Verification items for the finished model (mm, model axes). A direction names the side the tool comes from. Give positions to 0.01 mm unless a question says otherwise; leave off trailing zeros. Write each loop counter-clockwise with the first axis right and the second up, starting at its lowest first coordinate (ties: lowest second). Pieces come first, ordered by that corner, then holes. Notation, with made-up numbers: (64, 34.5) -> (123, 34.5) arc R27 cw to (123, 59.5) -> close; hole circle Ø5 at (38.25, 64). An arc over 180 degrees is marked (long way). Use one line per item in the form item = value. Start each with the question number.
(1) Section check A-A, the plane x = -3.25. Record the cut outline in (y, z).
(2) Set-up check for faces 1 (the face through (-8.248, 11, -5)), 2 (the face through (2.692, -16.756, -3.409)), 3 (the face through (-11.187, -12.966, 1.479)): record each of +Z, -Z, +X, -X, +Y, -Y from which the full face is reachable in a straight line by a thin tool's end or side.
(3) Section check C-C, the plane y = 4.5. Record the cut outline in (x, z), plus the area to 3 significant figures.
(4) Depth check by flat-ended pin: pin 1 Ø1 at (x, y) = (-7, 57.5) entering from -Z; pin 2 Ø6.5 at (x, y) = (5.78, 63.88) entering from -Z; pin 3 Ø3 at (y, z) = (15.5, -3.5) entering from -X; pin 4 Ø3 at (y, z) = (0.5, -2.5) entering from +X. Enter the tip coordinate at first touch or a pass-through.
(5) Section check D-D, the plane z = 2. Record the cut outline in (x, y), plus the area to 3 significant figures.
(6) Section check B-B, the plane z = -4.5. Record the cut outline in (x, y), plus the area to 3 significant figures.
(7) Scan lines: L1, parallel to Z at x = -1, y = -17; L2, parallel to X at y = 3.5, z = -7.75; L3, parallel to X at y = -1.5, z = 1.75. Record each from-to range of solid material in increasing order.
(8) Release check for a two-part mould opening along X. For faces 4 (the face through (5.24, 61.44, 1.48)), 5 (the face through (-6.879, 10, -3)), 6 (the face through (1.24, -17.16, -4.93)), 7 (the face through (-4, -8, -10)) record: pulls with the +X half, pulls with the -X half, needs draft (parallel to the pull), parting line crosses it, or undercut.
from build123d import *

# Parameters (mm, degrees)
EXTRUDE_4_DEPTH     = 3
SKETCH_2_R          = 2.5
CUT_EXTRUDE_1_DEPTH = 72.936469634
EXTRUDE_6_DEPTH     = 10


with BuildPart() as part:
    # 草图1 → 凸台-拉伸4 (new body)
    with BuildSketch(Plane.XY):
        with BuildLine():
            ThreePointArc((11.999755772, 64.190702015), (7.19287537, 69.699227744), (0.441332655, 66.894477154))
            Line((0.441332655, 66.894477154), (-16.87917542, 36.894477154))
            Line((-16.87917542, 36.894477154), (-16.87917542, -3.105522846))
            Line((-16.87917542, -3.105522846), (-5.332170037, -23.105522846))
            Line((-5.332170037, -23.105522846), (9.992741519, -33.105522846))
            Line((9.992741519, -33.105522846), (11.999755772, -30.029791253))
            Line((11.999755772, -30.029791253), (-6.87917542, -3.105522846))
            Line((-6.87917542, -3.105522846), (-6.87917542, 14.190702015))
            Line((-6.87917542, 14.190702015), (-6.87917542, 24.190702015))
            Line((-6.87917542, 24.190702015), (10.114332844, 34.190702015))
            Line((10.114332844, 34.190702015), (11.999755772, 64.190702015))
        make_face()
    extrude(amount=EXTRUDE_4_DEPTH)

    # 草图2 → 切除-拉伸1 (cut, through all)
    with BuildSketch(Plane.XY):
        with Locations((5.784422652, 63.881230161)):
            Circle(SKETCH_2_R)
    extrude(amount=CUT_EXTRUDE_1_DEPTH, mode=Mode.SUBTRACT)

    # 草图6 → 凸台-拉伸6 (add)
    with BuildSketch(Plane(origin=(0, 0, 0), x_dir=(-1, 0, 0), z_dir=(0, 0, -1))):
        Polygon((6.87917542, 24.190702015), (8.248400541, 24.190702015), (8.248400541, -3.145484966), (-10.996248645, -31.567657049), (-11.999755772, -30.029791253), (6.87917542, -3.105522846), align=None)
    extrude(amount=EXTRUDE_6_DEPTH)


solid = part.part
Completed:
q1.outline = (-24.46, 0) -> (-10.53, 0) -> (-10.53, -10) -> (-8.28, -10) -> (-8.28, 3) -> (-24.46, 3) -> close; (26.33, 0) -> (60.5, 0) -> (60.5, 3) -> (26.33, 3) -> close
q2.face_1 = -Z, -X, +Y, -Y
q2.face_2 = +Z, -Z, +X
q2.face_3 = +Z, -Z, -X, -Y
q3.outline = (-16.88, 0) -> (-8.25, 0) -> (-8.25, -10) -> (-6.88, -10) -> (-6.88, 3) -> (-16.88, 3) -> close
q3.area = 43.7 mm²
q4.pin_1 = through
q4.pin_2 = 0
q4.pin_3 = -8.25
q4.pin_4 = -6.88
q5.outline = (-16.88, -3.11) -> (-5.33, -23.11) -> (9.99, -33.11) -> (12, -30.03) -> (-6.88, -3.11) -> (-6.88, 24.19) -> (10.11, 34.19) -> (12, 64.19) arc R6.26 ccw to (0.44, 66.89) -> (-16.88, 36.89) -> close; hole circle Ø5 at (5.78, 63.88)
q5.area = 1,420 mm²
q6.outline = (-8.25, -3.15) -> (11, -31.57) -> (12, -30.03) -> (-6.88, -3.11) -> (-6.88, 24.19) -> (-8.25, 24.19) -> close
q6.area = 85.3 mm²
q7.L1 = 0 to 3
q7.L2 = -8.25 to -6.88
q7.L3 = -16.88 to -6.88
q8.face_4 = undercut
q8.face_5 = pulls with the +X half
q8.face_6 = pulls with the -X half
q8.face_7 = needs draft
